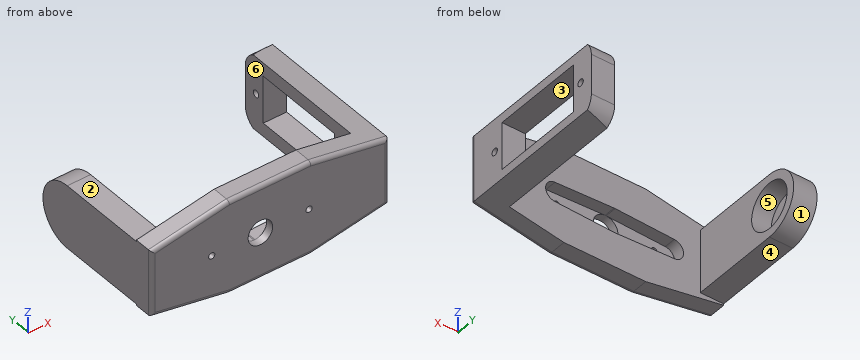
```python
from build123d import *

# Parameters (mm, degrees)
SKETCH_1_W          = 61
SKETCH_1_H          = 24
EXTRUDE_1_DEPTH     = 5
SKETCH_2_W          = 16.198202564
SKETCH_2_H          = 31.099101282
SKETCH_2_R          = 5.9
EXTRUDE_2_DEPTH     = 6
SKETCH_8_R          = 5.9
EXTRUDE_4_DEPTH     = 1
FILLET_1_RADIUS     = 8.099101282
FILLET_1_LENGTH     = 6
SKETCH_3_W          = 20.26798367
SKETCH_3_H          = 35.075185683
SKETCH_3_R          = 0.9
SKETCH_3_W_2        = 12.2
SKETCH_3_H_2        = 23.8
EXTRUDE_3_DEPTH     = 6
FILLET_2_R          = 5
CHAMFER_1_SIZE      = 3.526539614
CHAMFER_1_SIZE_2    = 20
FILLET_4_R          = 1
CUT_EXTRUDE_1_DEPTH = 3
SKETCH_5_R          = 3.15
SKETCH_5_R_2        = 0.8
CUT_EXTRUDE_2_DEPTH = 2.4


with BuildPart() as part:
    # 草图1 → 凸台-拉伸1 (new body)
    with BuildSketch(Plane(origin=(0, 0, 0), x_dir=(1, 0, 0), z_dir=(0, 1, 0))):
        with Locations((2.5, 0)):
            Rectangle(SKETCH_1_W, SKETCH_1_H)
    extrude(amount=EXTRUDE_1_DEPTH)

    # 草图2 → 凸台-拉伸2 (add)
    with BuildSketch(Plane.ZY.offset(28)):
        with Locations((0, 20.549550641)):
            Rectangle(SKETCH_2_W, SKETCH_2_H)
        with Locations((0, 28)):
            Circle(SKETCH_2_R, mode=Mode.SUBTRACT)
    extrude(amount=-EXTRUDE_2_DEPTH)

    # 草图8 → 凸台-拉伸4 (add)
    with BuildSketch(Plane.ZY.offset(28)):
        with Locations((0, 28)):
            Circle(SKETCH_8_R)
    extrude(amount=-EXTRUDE_4_DEPTH)

    # 圆角1: full round fillet: the end face becomes a half cylinder, R = half its width
    fillet_1_face = Plane((-25, 36.099101282, 0), x_dir=(-1, 0, 0), z_dir=(0, 1, 0))  # on the end face: x along it, z out of the body
    fillet_1_slab = fillet_1_face.offset(-FILLET_1_RADIUS / 2) * Box(FILLET_1_LENGTH, 2 * FILLET_1_RADIUS, FILLET_1_RADIUS, mode=Mode.PRIVATE)  # the body's end, R deep
    fillet_1_round = Plane((-25, 28, 0), x_dir=(0, 1, 0), z_dir=(-1, 0, 0)) * Cylinder(FILLET_1_RADIUS, FILLET_1_LENGTH, mode=Mode.PRIVATE)  # its axis R under the face
    add(fillet_1_slab - fillet_1_round, mode=Mode.SUBTRACT)

    # 草图3 → 凸台-拉伸3 (add)
    with BuildSketch(Plane(origin=(33, 0, 0), x_dir=(0, 0, -1), z_dir=(1, 0, 0))):
        with Locations((0, 22.537592842)):
            Rectangle(SKETCH_3_W, SKETCH_3_H)
        with Locations((0, 7.9)):
            Circle(SKETCH_3_R, mode=Mode.SUBTRACT)
        with Locations(Location((0, 36.5, 0), (0, 0, 180))):
            Circle(SKETCH_3_R, mode=Mode.SUBTRACT)
        with Locations((0, 22.2)):
            Rectangle(SKETCH_3_W_2, SKETCH_3_H_2, mode=Mode.SUBTRACT)
    extrude(amount=-EXTRUDE_3_DEPTH)

    # 圆角2
    fillet_2_edges = [part.edges().sort_by_distance(p)[0] for p in [
        (30, 40.075185683, 10.133991835),
        (30, 40.075185683, -10.133991835),
    ]]
    fillet(fillet_2_edges, radius=FILLET_2_R)

    # 倒角1
    # the kernel refuses this chamfer: 20, 3.526539614 mm, written as the material it takes off along each edge
    with BuildSketch(Plane(origin=(33, -51.970775928, -12), x_dir=(0.21013876076743143, 0, 0.9776715712462587), z_dir=(0, 1, 0))) as chamfer_1_piece_1:
        Polygon((CHAMFER_1_SIZE * 0.977671571293, -CHAMFER_1_SIZE * 0.210138760778), (-CHAMFER_1_SIZE_2 * 0.210138760767, -CHAMFER_1_SIZE_2 * 0.977671571246), (0, 0), align=None)
    extrude(amount=108.941551857, mode=Mode.SUBTRACT)
    with BuildSketch(Plane(origin=(-28, -51.970775928, -12), x_dir=(0.9999776716360547, 0, -0.006682531656102014), z_dir=(0, 1, 0))) as chamfer_1_piece_2:
        Polygon((CHAMFER_1_SIZE_2 * 0.999977671636, -CHAMFER_1_SIZE_2 * 0.0066825316561), (-CHAMFER_1_SIZE * 0.00668253165642, -CHAMFER_1_SIZE * 0.999977671684), (0, 0), align=None)
    extrude(amount=108.941551857, mode=Mode.SUBTRACT)
    with BuildSketch(Plane(origin=(33, -51.970775928, 12), x_dir=(0.21013876076743124, 0, -0.9776715712462587), z_dir=(0, 1, 0))) as chamfer_1_piece_3:
        Polygon((CHAMFER_1_SIZE * 0.977671571293, CHAMFER_1_SIZE * 0.210138760778), (-CHAMFER_1_SIZE_2 * 0.210138760767, CHAMFER_1_SIZE_2 * 0.977671571246), (0, 0), align=None)
    extrude(amount=108.941551857, mode=Mode.SUBTRACT)
    with BuildSketch(Plane(origin=(-28, -51.970775928, 12), x_dir=(0.9999776716360547, 0, 0.006682531656101331), z_dir=(0, 1, 0))) as chamfer_1_piece_4:
        Polygon((CHAMFER_1_SIZE_2 * 0.999977671636, CHAMFER_1_SIZE_2 * 0.0066825316561), (-CHAMFER_1_SIZE * 0.00668253165642, CHAMFER_1_SIZE * 0.999977671684), (0, 0), align=None)
    extrude(amount=108.941551857, mode=Mode.SUBTRACT)

    # 圆角4
    fillet_4_edges = [part.edges().sort_by_distance(p)[0] for p in [
        (2.5, 0, -12),
        (-28, 0, 0),
        (33, 0, 0),
        (2.5, 0, 12),
        (-18, 0, -10.236730193),
        (-18, 0, 10.236730193),
        (23, 0, 10.236730193),
        (23, 0, -10.236730193),
    ]]
    fillet(fillet_4_edges, radius=FILLET_4_R)

    # 草图4 → 切除-拉伸1 (cut)
    with BuildSketch(Plane(origin=(-24, 5, 6), x_dir=(-1, 0, 0), z_dir=(0, -1, 0))):
        with BuildLine():
            Line((-23.865345259, 9.147120605), (-8.68757668, 8.497714766))
            ThreePointArc((-8.68757668, 8.497714766), (-6.294445522, 6), (-8.68757668, 3.502285234))
            Line((-8.68757668, 3.502285234), (-23.865345259, 2.852879395))
            ThreePointArc((-23.865345259, 2.852879395), (-27.15, 6), (-23.865345259, 9.147120605))
        make_face()
    cut_extrude_1 = extrude(amount=CUT_EXTRUDE_1_DEPTH, mode=Mode.SUBTRACT)

    # 镜向1: 切除-拉伸1 across plane
    add(cut_extrude_1.mirror(Plane(origin=(0, 0, 0), x_dir=(0, 0, 1), z_dir=(1, 0, 0))), mode=Mode.SUBTRACT)

    # 草图5 → 切除-拉伸2 (cut)
    with BuildSketch(Plane(origin=(0, 2, 0), x_dir=(1, 0, 0), z_dir=(0, 1, 0))):
        with Locations(Location((0, 0, 0), (0, 0, 270))):
            Circle(SKETCH_5_R)
        with Locations(Location((-12.5, 0, 0), (0, 0, 270))):
            Circle(SKETCH_5_R_2)
        with Locations(Location((12.5, 0, 0), (0, 0, 270))):
            Circle(SKETCH_5_R_2)
    extrude(amount=-CUT_EXTRUDE_2_DEPTH, mode=Mode.SUBTRACT)


solid = part.part
```
Geometry: final body of the model. Coordinates: model frame, mm. Face numbers are marked on the shaded views. A direction names the side the tool comes from. Round coordinates to 2 decimals unless told otherwise and drop trailing zeros. Loops run counter-clockwise (first coordinate to the right, second up) from the corner with the lowest first, then second, coordinate; pieces in that order, holes last.
Item 1: Section A-A, the plane y = 7.9. Output: boundary loops of the cut face in (x, z).
Checked values:
outline: (-28, -8.1) - (-22, -8.1) - (-22, 8.1) - (-28, 8.1) - close; (27, -9.53) - (33, -8.47) - (33, -0.9) - (27, -0.9) - close; (27, 0.9) - (33, 0.9) - (33, 8.47) - (27, 9.53) - close
Item 2: Contact query for flat-ended pins moving along their axis: P1, Ø12, axis at x = -11, y = 13.5, coming from the +Z side; P2, Ø6.5, axis at x = 30, y = 17.5, coming from the -Z side; P3, Ø7, axis at x = 5.5, z = 0.5, coming from the +Y side; P4, Ø3, axis at x = -25.5, y = 20, coming from the +Z side. Output: stop coordinate, or through.
Checked values:
P1: passes through
P2: stops at z = -9.53
P3: stops at y = 5
P4: stops at z = 8.1
Item 3: Section C-C, the plane z = 0. State how many separate pieces and enclosed holes the cut face has, plus the area to 3 significant figures.
Checked values:
separate pieces: 7
enclosed holes: 0
area: 353 mm2
Item 4: Section B-B, the plane z = -4.5. Output: boundary loops of the cut face in (x, y), plus the area to 3 significant figures.
Checked values:
outline: (-28, 1) arc R1 ccw to (-27, 0) - (32, 0) arc R1 ccw to (33, 1) - (33, 10.3) - (27, 10.3) - (27, 5) - (-22, 5) - (-22, 24.18) - (-27, 24.18) - (-27, 31.82) - (-22, 31.82) - (-22, 34.73) - (-28, 34.73) - close; (27, 34.1) - (33, 34.1) - (33, 40.08) - (27, 40.08) - close
area: 512 mm2
Item 5: Mould query, pull axis Y, two halves, no side actions, for the marked faces 1, 2 and 3. Classes: released by +Y, released by -Y, zero draft, split by the parting line, or undercut.
Checked values:
face 1: released by +Y
face 2: zero draft
face 3: undercut
Item 6: Reachability of the marked faces 4, 5 and 6 from +Z, -Z, +X, -X, +Y, -Y: full face, straight path, thin tool, end or side. Return the list, or none.
Checked values:
face 4: -Z, -X, +Y
face 5: +X
face 6: +Z, -Z, +Y
Item 7: Section D-D, the plane y = 20. Output: boundary loops of the cut face in (x, z), plus the area to 3 significant figures.
Checked values:
outline: (-28, -8.1) - (-22, -8.1) - (-22, 8.1) - (-28, 8.1) - close; (27, -9.53) - (33, -8.47) - (33, -6.1) - (27, -6.1) - close; (27, 6.1) - (33, 6.1) - (33, 8.47) - (27, 9.53) - close
area: 132 mm2
Item 8: Line query: L1, parallel to X at y = 1, z = 0; L2, parallel to Z at x = 0, y = 1.65; L3, parallel to X at y = 21.5, z = 6.75. Output: solid intervals per line, ascending.
Checked values:
L1: x = -28 to -13.3, -11.7 to -3.15, 3.15 to 11.7, 13.3 to 33
L2: z = -12 to -3.15, 3.15 to 12
L3: x = -28 to -22, 27 to 33
